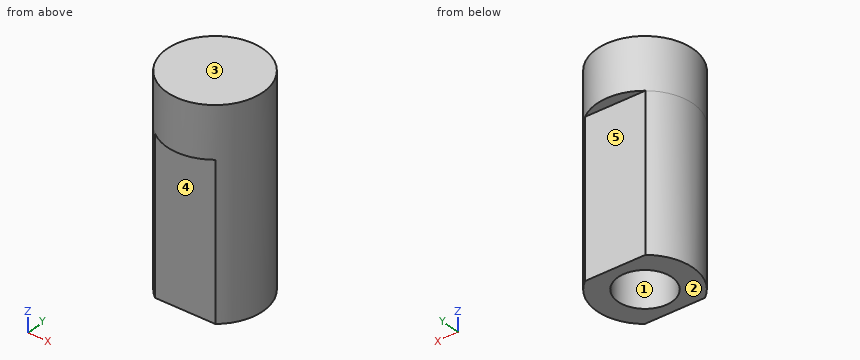
```python
from build123d import *
from build123d.topology import SkipClean

# Parameters (mm, degrees)
EXTRUDE1_DEPTH              = 30.48
EXTRUDE2_START              = 25.4
SKETCH2_R                   = 9.525
EXTRUDE2_DEPTH              = 25.4
F_1_2_13_TAPPED_HOLE1_D     = 10.71626
F_1_2_13_TAPPED_HOLE1_DEPTH = 31.25978
F_1_2_13_TAPPED_HOLE1_TIP   = 3.219489309
SKETCH6_R                   = 9.525
CUT_EXTRUDE1_DEPTH          = 15.24


with BuildPart() as part:
    # Sketch1 → Extrude1 (new body)
    with BuildSketch(Plane.XY):
        with BuildLine():
            Line((-5.880525147, 7.493), (5.880525147, 7.493))
            ThreePointArc((5.880525147, 7.493), (9.525, 0), (5.880525147, -7.493))
            Line((5.880525147, -7.493), (-5.880525147, -7.493))
            ThreePointArc((-5.880525147, -7.493), (-9.525, 0), (-5.880525147, 7.493))
        make_face()
    extrude(amount=-EXTRUDE1_DEPTH)

    # Sketch2 → Extrude2 (add)
    with SkipClean():  # the faces are left unmerged after this step: merging them gives an invalid solid
        with BuildSketch(Plane.XY.offset(EXTRUDE2_START)):
            Circle(SKETCH2_R)
        extrude(amount=-EXTRUDE2_DEPTH)

    # 1/2-13 Tapped Hole1
    with Locations(Plane(origin=(0, 0, -30.48), x_dir=(-1, 0, 0), z_dir=(0, 0, -1))):
        with Locations((0, 0)):
            Hole(F_1_2_13_TAPPED_HOLE1_D / 2, depth=F_1_2_13_TAPPED_HOLE1_DEPTH)
            with Locations((0, 0, -(F_1_2_13_TAPPED_HOLE1_DEPTH + F_1_2_13_TAPPED_HOLE1_TIP / 2))):  # 118° drill point
                Cone(0, F_1_2_13_TAPPED_HOLE1_D / 2, F_1_2_13_TAPPED_HOLE1_TIP, mode=Mode.SUBTRACT)

    # Sketch6 → Cut-Extrude1 (cut)
    with SkipClean():  # the faces are left unmerged after this step: merging them gives an invalid solid
        with BuildSketch(Plane.XY.offset(25.4)):
            Circle(SKETCH6_R)
        extrude(amount=-CUT_EXTRUDE1_DEPTH, mode=Mode.SUBTRACT)


solid = part.part
```
Verification items for the finished model (mm, model axes). Face numbers are marked on the shaded views. A direction names the side the tool comes from. Round coordinates to 2 decimals unless told otherwise and drop trailing zeros. Write each loop counter-clockwise with the first axis right and the second up, starting at its lowest first coordinate (ties: lowest second). Pieces come first, ordered by that corner, then holes. Notation, with made-up numbers: (16.5, 32.25) - (36.5, 32.25) arc R16 ccw to (36.5, 52.25) - close; hole circle Ø1 at (-5.5, 8). An arc over 180 degrees is marked (long way). Answer as a JSON object with one key per item and string values. Group by question number.
Q1. Tool access check on the marked faces 3, 4 and 5. Record the directions out of +Z, -Z, +X, -X, +Y, -Y that give a thin tool (end or side, any length) a straight path to the whole face; none if there is none.
Q2. Go/stop test with flat-tipped pins: pin 1 Ø3.5 at (x, z) = (2, -21) entering from +Y; pin 2 Ø8 at (y, z) = (-1.5, 0.5) entering from +X (3 decimals); pin 3 Ø1.6 at (x, y) = (2, -8.5) entering from -Z; pin 4 Ø6 at (y, z) = (5.5, -11) entering from -X. Record where each tip stops, or that it passes through.
Q3. Section check A-A, the plane y = 7. Enter the section's corners in (x, z).
Q4. Mould release check, pull along X, two halves, no side actions. Record for the marked faces 1 and 2: released by +X, released by -X, zero draft, split by the parting line, or undercut.
Q5. Section check B-B, the plane x = -6.75. Enter the section's corners in (y, z), plus the area to 3 significant figures.
Q6. Thickness scan on line 1 (X direction, y = 0, z = -15) (3 decimals); line 2 (Y direction, x = 0, z = -17); line 3 (Y direction, x = 2.5, z = -15). Record the ranges inside material, lowest first.
Found:
{
 "1": {"face 3": "+Z, +X, -X, +Y, -Y", "face 4": "-Z, +X, -X, -Y", "face 5": "-Z, +X, -X, +Y"},
 "2": {"pin 1": "stops at y = 7.49", "pin 2": "stops at x = 9.525", "pin 3": "stops at z = 0", "pin 4": "stops at x = -9.19"},
 "3": {"outline": "(-6.46, -30.48) - (6.46, -30.48) - (6.46, 10.16) - (-6.46, 10.16) - close"},
 "4": {"face 1": "undercut", "face 2": "zero draft"},
 "5": {"outline": "(-6.72, -30.48) - (6.72, -30.48) - (6.72, 10.16) - (-6.72, 10.16) - close", "area": "546 mm^2"},
 "6": {"line 1": "x = -9.525 to -5.358, 5.358 to 9.525", "line 2": "y = -7.49 to -5.36, 5.36 to 7.49", "line 3": "y = -7.49 to -4.74, 4.74 to 7.49"}
}
